The listing builds one solid part. Answer for the finished solid, in the listing's coordinates (mm). A direction names the side the tool comes from. Coordinates: 2 decimals unless noted, no trailing zeros. Loops run counter-clockwise (first coordinate to the right, second up) from the corner with the lowest first, then second, coordinate; pieces in that order, holes last. Notation, with made-up numbers: (5.25, 37) -> (25.25, 37) arc R22 cw to (25.25, 43) -> close; hole circle Ø4 at (25, 35). An arc over 180 degrees is marked (long way). Answer in a Markdown table with one row per item.
Autodesk Inventor part; units mm, degrees
ref_plane "YZ Plane" through (0, 0, 0) normal (1, 0, 0) x (0, 1, 0)
ref_plane "XZ Plane" through (0, 0, 0) normal (0, 1, 0) x (-1, 0, 0)
ref_plane "XY Plane" through (0, 0, 0) normal (0, 0, 1) x (1, 0, 0)
ref_plane "Arbeitsebene1" through (0, 0, 0) normal (0, 0, 1) x (1, 0, 0)
sketch "Skizze1" plane through (0, 0, 0) normal (0, 0, 1) x (1, 0, 0)
  circle A0 centre (-59.69, 23.2744) radius 1.6
  circle A1 centre (59.69, 23.2744) radius 1.6
  circle A2 centre (59.69, -23.7156) radius 1.6
  circle A3 centre (-59.69, -23.7156) radius 1.6
  circle A4 centre (-59.69, 23.2744) radius 3
  circle A5 centre (59.69, 23.2744) radius 3
  circle A6 centre (59.69, -23.7156) radius 3
  circle A7 centre (-59.69, -23.7156) radius 3
  point P0 (0, 0)
  dimension "d0" = 6
  dimension "d1" = 6
  dimension "d2" = 6
  dimension "d3" = 6
extrude "Extrusion1" add sketch "Skizze1" along normal blind 3
ref_plane "Arbeitsebene2" through (0, 0, 0) normal (0, 0, 1) x (1, 0, 0)
sketch "Skizze2" plane through (0, 0, 0) normal (0, 0, 1) x (1, 0, 0)
  line L0 (-30.04, 15.6244) -> (-27.04, 15.6244)
  line L1 (-27.04, -19.3756) -> (-30.04, -19.3756)
  line L2 (-20.04, 0.6244) -> (-20.04, -4.3756)
  line L3 (-37.04, -4.3756) -> (-37.04, 0.6244)
  line L4 (-1.04, 9.6244) -> (3.96, 9.6244)
  line L5 (3.96, -8.3756) -> (-1.04, -8.3756)
  line L6 (10.96, 0.6244) -> (10.96, -4.3756)
  line L7 (-8.04, -4.3756) -> (-8.04, 0.6244)
  line L8 (40.96, -1.3756) -> (53.96, -1.3756)
  line L9 (53.96, -1.3756) -> (53.96, -4.3756)
  line L10 (53.96, -4.3756) -> (40.96, -4.3756)
  line L11 (40.96, -4.3756) -> (40.96, -1.3756)
  line L12 (-8.04, 0.6244) -> (-1.04, 0.6244)
  line L13 (3.96, 0.6244) -> (10.96, 0.6244)
  line L14 (3.96, 9.6244) -> (3.96, 0.6244)
  line L15 (3.96, -4.3756) -> (3.96, -8.3756)
  line L16 (10.96, -4.3756) -> (3.96, -4.3756)
  line L17 (-1.04, -4.3756) -> (-8.04, -4.3756)
  line L18 (-1.04, -8.3756) -> (-1.04, -4.3756)
  line L19 (-1.04, 0.6244) -> (-1.04, 9.6244)
  line L20 (-37.04, 0.6244) -> (-30.04, 0.6244)
  line L21 (-27.04, 0.6244) -> (-20.04, 0.6244)
  line L22 (-27.04, 15.6244) -> (-27.04, 0.6244)
  line L23 (-27.04, -4.3756) -> (-27.04, -19.3756)
  line L24 (-30.04, -19.3756) -> (-30.04, -4.3756)
  line L25 (-30.04, 0.6244) -> (-30.04, 15.6244)
  line L26 (-20.04, -4.3756) -> (-27.04, -4.3756)
  line L27 (-30.04, -4.3756) -> (-37.04, -4.3756)
  line L28 (-66.04, -24.3506) -> (-66.04, 23.2744)
  line L29 (-59.69, 29.6244) -> (59.69, 29.6244)
  point P0 (0, 0)
  dimension "d6" = 3
  dimension "d7" = 7
  dimension "d8" = 7
  dimension "d9" = 7
  dimension "d10" = 7
  dimension "d11" = 3
  dimension "d12" = 15
  dimension "d13" = 15
  dimension "d14" = 15
  dimension "d15" = 15
  dimension "d16" = 5
  dimension "d17" = 29
  dimension "d18" = 14
  dimension "d19" = 20
  dimension "d20" = 18
  dimension "d21" = 7
  dimension "d22" = 7
  dimension "d23" = 12
  dimension "d24" = 5
  dimension "d25" = 13
  dimension "d26" = 30
  dimension "d27" = 31
extrude "Extrusion2" add sketch "Skizze2" along normal up to surface (3 mm away)
sketch "Skizze3" plane through (-8.04, 0.6244, 3) normal (0, 0, 1) x (1, 0, 0)
  line L0 (-59.65, 30.65) -> (77.33, 30.65)
  line L1 (77.33, 30.65) -> (77.33, -32.34)
  line L2 (77.33, -32.34) -> (-59.65, -32.34)
  line L3 (-59.65, -32.34) -> (-59.65, 30.65)
  circle A0 centre (67.73, 22.65) radius 1.6
  circle A1 centre (-51.65, 22.65) radius 1.6
  circle A2 centre (-51.65, -24.34) radius 1.6
  circle A3 centre (67.73, -24.34) radius 1.6
  point P0 (8.04, -0.6244)
  dimension "d31" = 8
  dimension "d32" = 8
  dimension "d33" = 8
  dimension "d34" = 8
extrude "Extrusion3" add sketch "Skizze3" along normal blind 3
fillet "Rundung1" radius 3.75 4 edges at (-62.69, -23.7156, 3) (56.69, -23.7156, 3) (56.69, 23.2744, 3) (-62.69, 23.2744, 3)
sketch "Skizze5" plane through (-8.04, 0.6244, 6) normal (0, 0, 1) x (1, 0, 0)
  circle A0 centre (67.73, 22.65) radius 1.6
  circle A1 centre (67.73, 22.65) radius 6
  circle A2 centre (67.73, -24.34) radius 6
  circle A3 centre (-51.65, 22.65) radius 1.6
  circle A4 centre (-51.65, 22.65) radius 6
  circle A5 centre (-51.65, -24.34) radius 6
  circle A6 centre (-51.65, -24.34) radius 1.6
  circle A7 centre (67.73, -24.34) radius 1.6
  point P0 (8.04, -0.6244)
  dimension "d44" = 12
  dimension "d45" = 12
  dimension "d46" = 12
  dimension "d47" = 12
extrude "Extrusion5" cut sketch "Skizze5" against normal blind 2
sketch "Skizze6" plane through (-67.69, 31.2744, 3) normal (0, 1, 0) x (1, 0, 0)
  line L0 (0, 0) -> (136.98, 0)
  line L1 (59.98, 0) -> (77.98, 0)
  line L2 (77.98, 0) -> (77.98, -1.5)
  line L3 (77.98, -1.5) -> (59.98, -1.5)
  line L4 (59.98, -1.5) -> (59.98, 0)
  line L5 (136.98, 0) -> (136.98, -3)
  point P0 (67.69, 3)
  dimension "d50" = 1.5
  dimension "d51" = 18
  dimension "d52" = 59
extrude "Extrusion6" cut sketch "Skizze6" against normal blind 4
move faces "Verschieben1" translate (0, 0, 2.5) faces at (4.29, 29.9411, 4.5)
sketch "Skizze7" plane through (-8.04, 0.6244, 6) normal (0, 0, 1) x (1, 0, 0)
  line L0 (-59.65, 30.65) -> (-59.65, -32.34)
  line L1 (-59.65, -32.34) -> (77.33, -32.34)
  line L2 (0.33, 30.65) -> (-59.65, 30.65)
  line L3 (77.33, -32.34) -> (77.33, 30.65)
  line L4 (77.33, 30.65) -> (18.33, 30.65)
  line L5 (-54.65, -32.34) -> (72.33, -32.34)
  line L6 (77.33, -27.34) -> (77.33, 25.65)
  line L7 (-59.65, 25.65) -> (-59.65, -27.34)
  line L8 (0.33, 26.65) -> (18.33, 26.65)
  line L9 (18.33, 30.65) -> (18.33, 26.65)
  line L10 (18.33, 26.65) -> (0.33, 26.65)
  line L11 (0.33, 26.65) -> (0.33, 30.65)
  line L12 (72.33, 30.65) -> (18.33, 30.65)
  line L13 (0.33, 30.65) -> (-54.65, 30.65)
  line L14 (0.33, 30.65) -> (0.33, 26.65)
  arc A0 (-59.65, -27.34) -> (-54.65, -32.34) centre (-54.65, -27.34) ccw
  arc A1 (-54.65, 30.65) -> (-59.65, 25.65) centre (-54.65, 25.65) ccw
  arc A2 (72.33, -32.34) -> (77.33, -27.34) centre (72.33, -27.34) ccw
  arc A3 (77.33, 25.65) -> (72.33, 30.65) centre (72.33, 25.65) ccw
  line L15 (-59.65, -27.34) -> (-59.65, -32.34)
  line L16 (-59.65, -32.34) -> (-54.65, -32.34)
  line L17 (-59.65, 30.65) -> (0.33, 30.65)
  line L18 (-59.65, 30.65) -> (-54.65, 30.65)
  line L19 (-59.65, 30.65) -> (-59.65, 25.65)
  line L20 (77.33, 30.65) -> (77.33, -32.34)
  line L21 (72.33, -32.34) -> (77.33, -32.34)
  line L22 (77.33, -32.34) -> (77.33, -27.34)
  line L23 (77.33, 25.65) -> (77.33, 30.65)
  line L24 (72.33, 30.65) -> (77.33, 30.65)
  point P0 (8.04, -0.6244)
  dimension "d58" = 4
  dimension "d59" = 4
  dimension "d60" = 5
equation "\"d1\" = d0"
equation "\"d2\" = d0"
equation "\"d3\" = d0"
equation "\"d7\" = d8"
equation "\"d9\" = d8"
equation "\"d10\" = d7"
equation "\"d14\" = d12"
equation "\"d15\" = d13"
equation "\"d21\" = d7"
equation "\"d22\" = d7"
equation "\"d32\" = d31"
equation "\"d33\" = d32"
equation "\"d34\" = d33"
equation "\"d45\" = d44"
equation "\"d46\" = d44"
equation "\"d47\" = d46"
properties part number "case_bot"
Item 1: Determine the mould class of faces 1 (the face through (39, 31.274, 4)), 2 (the face through (61, -25, 4)), 3 (the face through (69.29, 0, 4)) for opening direction X: +X half, -X half, draft (parallel to the pull), parting line (faces both ways), or undercut.
Findings below:
| item | result |
|---|---|
| face 1 | draft |
| face 2 | undercut |
| face 3 | +X half |
Item 2: A cutting plane is placed at B-B, the plane y = 13. Determine the outline of the cut face in (x, z).
Findings below:
| item | result |
|---|---|
| outline | (-67.69, 3) -> (-30.04, 3) -> (-30.04, 0) -> (-27.04, 0) -> (-27.04, 3) -> (69.29, 3) -> (69.29, 6) -> (-67.69, 6) -> close |
Item 3: Find the intervals of material crossed by probe 1 along X at (y, z) = (-3, 1.5); probe 2 along Y at (x, z) = (59.69, 5.1); probe 3 along Y at (x, z) = (59.69, 1.3), in increasing order.
Findings below:
| item | result |
|---|---|
| probe 1 | x = -37.04 to -20.04, -8.04 to 10.96, 40.96 to 53.96 |
| probe 2 | y = -31.72 to -29.72, -17.72 to 17.27, 29.27 to 31.27 |
| probe 3 | y = -27.25 to -25.32, -22.12 to -20.18, 19.74 to 21.67, 24.87 to 26.81 |
Item 4: A cutting plane is placed at C-C, the plane y = -3. Determine the outline of the cut face in (x, z), plus the area to 3 significant figures.
Findings below:
| item | result |
|---|---|
| outline | (-67.69, 3) -> (-37.04, 3) -> (-37.04, 0) -> (-20.04, 0) -> (-20.04, 3) -> (-8.04, 3) -> (-8.04, 0) -> (10.96, 0) -> (10.96, 3) -> (40.96, 3) -> (40.96, 0) -> (53.96, 0) -> (53.96, 3) -> (69.29, 3) -> (69.29, 6) -> (-67.69, 6) -> close |
| area | 558 mm2 |
Item 5: A tool of negligible diameter and unlimited length cuts with its end or side. For faces 4 (the face through (-1.04, 5, 1)), 5 (the face through (40.96, -3, 1)), 6 (the face through (-29, 15.624, 1)), 7 (the face through (-58, 22, 4)), 8 (the face through (-27.04, -12, 1)), from which of +Z, -Z, +X, -X, +Y, -Y can it reach the whole face along a straight path? Write none if from no direction.
Findings below:
| item | result |
|---|---|
| face 4 | -Z, +Y |
| face 5 | -Z, +Y, -Y |
| face 6 | -Z, +X, -X, +Y |
| face 7 | +Z |
| face 8 | -Z, -Y |
Item 6: A cutting plane is placed at A-A, the plane x = -59.69. Determine the outline of the cut face in (y, z), plus the area to 3 significant figures.
Findings below:
| item | result |
|---|---|
| outline | (-31.72, 3) -> (-30.39, 3) arc R3.75 cw to (-26.72, 0) -> (-25.32, 0) -> (-25.32, 4) -> (-29.72, 4) -> (-29.72, 6) -> (-31.72, 6) -> close; (-22.12, 0) -> (-20.72, 0) arc R3.75 cw to (-17.04, 3) -> (16.6, 3) arc R3.75 cw to (20.27, 0) -> (21.67, 0) -> (21.67, 4) -> (17.27, 4) -> (17.27, 6) -> (-17.72, 6) -> (-17.72, 4) -> (-22.12, 4) -> close; (24.87, 0) -> (26.27, 0) arc R3.75 cw to (29.95, 3) -> (31.27, 3) -> (31.27, 6) -> (29.27, 6) -> (29.27, 4) -> (24.87, 4) -> close |
| area | 162 mm2 |
Item 7: A cutting plane is placed at D-D, the plane y = 5. Determine the outline of the cut face in (x, z), plus the area to 3 significant figures.
Findings below:
| item | result |
|---|---|
| outline | (-67.69, 3) -> (-30.04, 3) -> (-30.04, 0) -> (-27.04, 0) -> (-27.04, 3) -> (-1.04, 3) -> (-1.04, 0) -> (3.96, 0) -> (3.96, 3) -> (69.29, 3) -> (69.29, 6) -> (-67.69, 6) -> close |
| area | 435 mm2 |
Item 8: Flat-ended cylindrical pins translate along their axes: pin 1 Ø0.9 at (x, z) = (50, 1) entering from -Y; pin 2 Ø0.9 at (y, z) = (-2.5, 2) entering from +X; pin 3 Ø3.5 at (x, z) = (1, 2) entering from +Y. Find the tip coordinate at first contact, or state that the pin passes through.
Findings below:
| item | result |
|---|---|
| pin 1 | stops at y = -4.38 |
| pin 2 | stops at x = 53.96 |
| pin 3 | stops at y = 27.27 |
